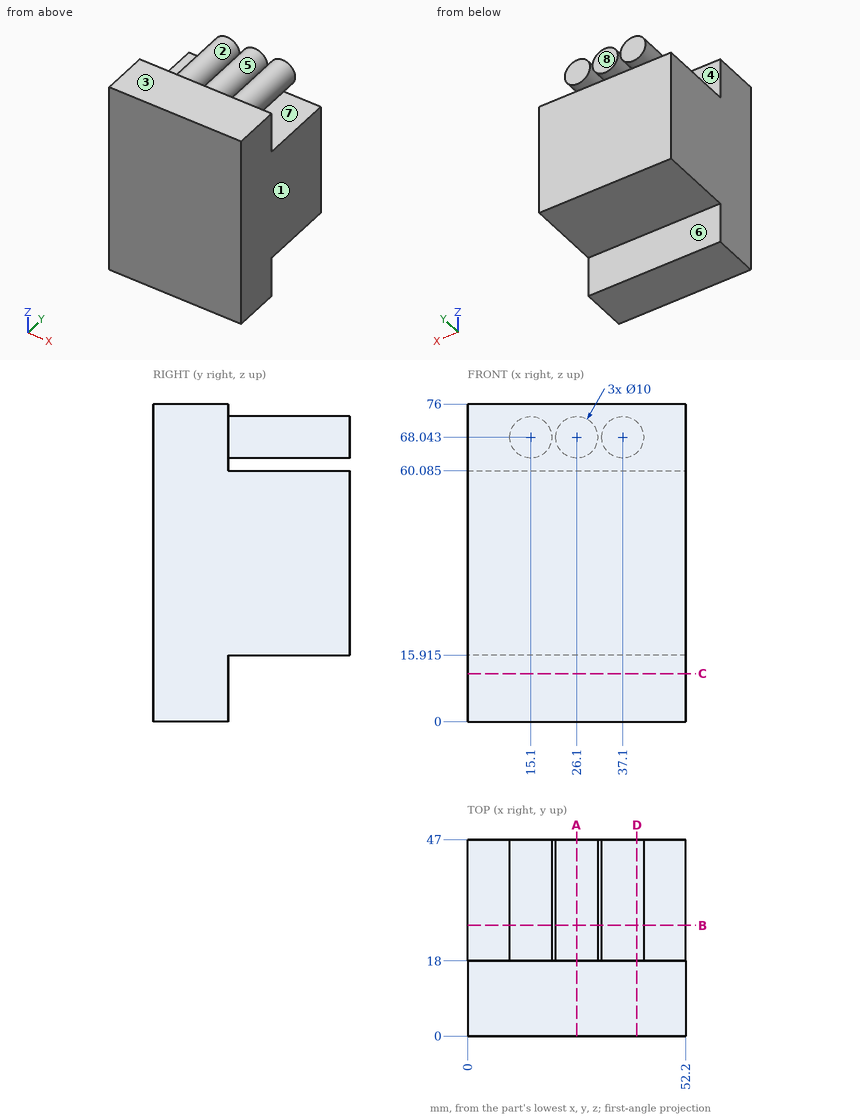
Answer from the drawing. Dimensions are ordinates in mm from the lowest x, y and z of the part. A direction names the side the tool comes from. Coordinates: 2 decimals unless noted, no trailing zeros. Write each loop counter-clockwise with the first axis right and the second up, starting at its lowest first coordinate (ties: lowest second). Pieces come first, ordered by that corner, then holes. Notation, with made-up numbers: (55, 17) -> (108, 17) arc R26 cw to (108, 40) -> close; hole circle Ø4 at (-2, 55.5). An arc over 180 degrees is marked (long way). One line per question, with ' | ' between items.
1. For a pull along Z with two mould halves and no side action, classify the marked faces 1, 2, 3 and 4 as released by +Z, released by -Z, zero draft, split by the parting line, or undercut.
Verdict:
face 1: zero draft | face 2: undercut | face 3: released by +Z | face 4: undercut
2. Section C-C (z = 11.5) is taken. Determine the outline of the cut face in (x, y).
Verdict:
outline: (0, 0) -> (52.2, 0) -> (52.2, 18) -> (0, 18) -> close
3. Section B-B (y = 26.5) is taken. Determine the outline of the cut face in (x, z) (1 decimal), and give its area (3 significant figures).
Verdict:
outline: (0, 15.9) -> (52.2, 15.9) -> (52.2, 60.1) -> (0, 60.1) -> close; circle Ø10 at (15.1, 68); circle Ø10 at (26.1, 68); circle Ø10 at (37.1, 68) | area: 2,540 mm^2
4. Which of the six approach directions +Z, -Z, +X, -X, +Y, -Y give full straight-line access (tool end or side, diameter ignored) to the marked faces 5, 6, 7 and 8?
Verdict:
face 5: +Y | face 6: -Z, +X, -X, +Y | face 7: +X, -X, +Y | face 8: +Z, -Z, +X, -X, +Y
5. Section D-D (x = 40.5) is taken. Determine the outline of the cut face in (y, z) (1 decimal), and give its area (3 significant figures).
Verdict:
outline: (0, 0) -> (18, 0) -> (18, 15.9) -> (47, 15.9) -> (47, 60.1) -> (18, 60.1) -> (18, 64.4) -> (47, 64.4) -> (47, 71.7) -> (18, 71.7) -> (18, 76) -> (0, 76) -> close | area: 2,860 mm^2
6. Section A-A (x = 26.1) is taken. Determine the outline of the cut face in (y, z) (1 decimal).
Verdict:
outline: (0, 0) -> (18, 0) -> (18, 15.9) -> (47, 15.9) -> (47, 60.1) -> (18, 60.1) -> (18, 63) -> (47, 63) -> (47, 73) -> (18, 73) -> (18, 76) -> (0, 76) -> close
7. Given pin 1 Ø2 at (x, y) = (39.5, 25.5) entering from +Z; pin 2 Ø8 at (x, y) = (15, 25) entering from +Z; pin 3 Ø12.5 at (x, z) = (35.5, 5.5) entering from +Y, each flat-ended and moving along its own axis, determine where each tip first touches the part or whether it passes through.
Verdict:
pin 1: stops at z = 72.84 | pin 2: stops at z = 73.04 | pin 3: stops at y = 18
8. Straight lines are drawn through the part: line 1 (X direction, y = 26, z = 70); line 2 (Z direction, x = 19.5, y = 35.5) (1 decimal); line 3 (Y direction, x = 12.5, z = 62.5). For each, find the intervals that lie inside material, in ascending order.
Verdict:
line 1: x = 10.5 to 19.7, 21.5 to 30.7, 32.5 to 41.7 | line 2: z = 15.9 to 60.1, 65.7 to 70.4 | line 3: y = 0 to 18
